Autodesk Inventor part; units mm, degrees
ref_plane "YZ Plane" through (0, 0, 0) normal (1, 0, 0) x (0, 1, 0)
ref_plane "XZ Plane" through (0, 0, 0) normal (0, 1, 0) x (-1, 0, 0)
ref_plane "XY Plane" through (0, 0, 0) normal (0, 0, 1) x (1, 0, 0)
sketch "Sketch1" plane through (0, 0, 0) normal (0, 0, 1) x (1, 0, 0)
  circle A0 centre (0, 0) radius 4.75
  circle A1 centre (0, 0) radius 5.4
  circle A2 centre (0, 0) radius 3.175
  dimension "d0" = 9.5
  dimension "d1" = 10.8
  dimension "d2" = 6.35
extrude "Extrusion1" add sketch "Sketch1" along normal blind 12 contours A2
extrude "Extrusion2" add sketch "Sketch1" against normal blind 80 contours A0
extrude "Extrusion3" add sketch "Sketch1" against normal blind 1.5 contours A1
sketch "Sketch2" plane through (0, 0, 0) normal (0, 0, -1) x (-1, 0, 0)
  circle A0 centre (0, 0) radius 3.175
  circle A1 centre (0, 0) radius 3.175
extrude "Extrusion4" add sketch "Sketch2" along normal blind 80
chamfer "Chamfer1" distance 0.3 angle 45 1 edges at (-3.175, 0, 12)
extrude "Extrusion5" add sketch "Sketch1" along normal blind 3 contours A0 | A1
equation "\"BendRadius\" = Thickness"
equation "\"BendReliefWidth\" = Thickness"
equation "\"BendReliefDepth\" = 0.5 * Thickness"
equation "\"CornerReliefSize\" = 4 * Thickness"
equation "\"MinimumRemnant\" = 2 * Thickness"
equation "\"TransitionRadius\" = BendRadius"
equation "\"JacobiRadiusSize\" = BendRadius"
equation "\"GapSize\" = Thickness"
properties part number "trục đai"
Verification items for the finished model (mm, model axes). A direction names the side the tool comes from. Round coordinates to 2 decimals unless told otherwise and drop trailing zeros. Write each loop counter-clockwise with the first axis right and the second up, starting at its lowest first coordinate (ties: lowest second). Pieces come first, ordered by that corner, then holes.
1. Section check A-A on y = 0. Enter the section's corners in (x, z) (3 decimals).
2. Gauge pin test, flat ends, axial feed: P1, Ø1, axis at x = 0, z = -42, coming from the +Y side; P2, Ø4, axis at y = -3, z = -54.5, coming from the +X side; P3, Ø1, axis at y = 1.5, z = -53.5, coming from the -X side. Record the tip position at first contact, or that the pin passes through.
3. Scan lines: L1, parallel to Z at x = 4.25, y = -2; L2, parallel to Z at x = 0, y = 5; L3, parallel to Y at x = 0.75, z = -21. Record each from-to range of solid material in increasing order.
4. Access from +Z, -Z, +X, -X, +Y, -Y to the whole of each face (thin tool, end or side, straight path). Record for faces 1 (the cylindrical face through (-0.69, 3.1, 7.29)), 2 (the cylindrical face through (2.192, -4.214, -40.2)), 3 (the flat face through (0, 0, 12)).
5. Section check C-C on z = -55. Enter the section's corners in (x, y), plus the area to 3 significant figures.
Answer:
1. outline: (-5.4, -1.5) - (-4.75, -1.5) - (-4.75, -80) - (4.75, -80) - (4.75, -1.5) - (5.4, -1.5) - (5.4, 3) - (3.175, 3) - (3.175, 11.7) - (2.875, 12) - (-2.875, 12) - (-3.175, 11.7) - (-3.175, 3) - (-5.4, 3) - close
2. P1: stops at y = 4.75
2. P2: stops at x = 4.64
2. P3: stops at x = -4.64
3. L1: z = -80 to 3
3. L2: z = -1.5 to 3
3. L3: y = -4.69 to 4.69
4. face 1: +Z
4. face 2: -Z
4. face 3: +Z, +X, -X, +Y, -Y
5. outline: circle Ø9.5 at (0, 0)
5. area: 70.9 mm2
